from build123d import *

# Parameters (mm, degrees)
F0_W     = 49.7
F0_H     = 1.5
F1_DEPTH = 142
F2_W     = 44.6868650615
F2_H     = 1.5
F3_DEPTH = 1
F4_R     = 0.99999


# Not quite as in the source:
# - a fillet or chamfer is up to 0.001 mm smaller than in the source, because OpenCascade refuses the exact size


with BuildPart() as f1:
    # F0 (on Front) → F1 (new body)
    with BuildSketch(Plane.XZ):
        with Locations((24.85, -0.75)):
            Rectangle(F0_W, F0_H)
        with Locations((-24.85, -0.75)):
            Rectangle(F0_W, F0_H)
        Polygon((49.7, -1.5), (0, -1.5), (0, -3), (50.5, -3), align=None)
        Polygon((0, -3), (0, -1.5), (-49.7, -1.5), (-50.5, -3), align=None)
    extrude(amount=F1_DEPTH)

    # F2 (on face) → F3 (join)
    with BuildSketch(Plane.XY):
        with Locations((-22.3434325308, -130.4639992552)):
            Rectangle(F2_W, F2_H)
        with Locations((22.3434325308, -130.4639992552)):
            Rectangle(F2_W, F2_H)
        with Locations((-22.3434325308, -126.9639992552)):
            Rectangle(F2_W, F2_H)
        with Locations((22.3434325308, -126.9639992552)):
            Rectangle(F2_W, F2_H)
        with Locations((-22.3434325308, -123.4639992552)):
            Rectangle(F2_W, F2_H)
        with Locations((22.3434325308, -123.4639992552)):
            Rectangle(F2_W, F2_H)
    extrude(amount=F3_DEPTH)

    # F4 (radius 1 in the source; OpenCascade refuses exactly that, so slightly less here)
    f4_edges = [f1.edges().sort_by_distance(p)[0] for p in [
        (-44.686865, -123.463999, 1),
        (-44.686865, -126.963999, 1),
        (-44.686865, -130.463999, 1),
        (44.686865, -123.463999, 1),
        (44.686865, -126.963999, 1),
        (44.686865, -130.463999, 1),
        (0, -142, 0),
    ]]
    fillet(f4_edges, radius=F4_R)


solid = f1.part
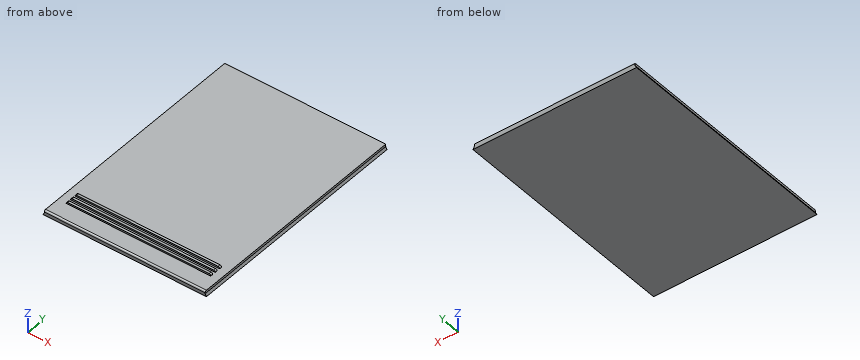
Geometry: final body of the model. Coordinates: model frame, mm. Coordinates: 2 decimals unless noted, no trailing zeros. Order: outer loops, then holes, each group sorted by start corner. A loop starts at its lowest first (then second) coordinate and runs counter-clockwise, first axis right, second up. Notation, with made-up numbers: M 17.25,42 L 72.25,42 A33 cw 72.25,75 Z; hole C 21.25,23.25 d7. An arc over 180 degrees is marked long. One line per question, with ' | ' between items. Start each with the question number.
Item 1: Pin query (flat end, axial travel): pin 1 Ø1.7 at (y, z) = (-79.5, -0.5) entering from -X; pin 2 Ø0.5 at (x, z) = (6.5, 0.5) entering from -Y; pin 3 Ø0.8 at (x, z) = (-6.5, 0.5) entering from +Y. Return the tip coordinate at first contact, or that it passes through.
Item 2: Cut plane B-B, the plane y = -68.5. Return the cut outline in (x, z).
Item 3: Ray query, probe 1 along Y at (x, z) = (25, 0.4); probe 2 along Z at (x, y) = (-19.5, -73.5); probe 3 along X at (y, z) = (-64, -0.9). Return the intervals inside material, ascending. Write a range as [from, to].
Item 4: Cut plane A-A, the plane x = 36.5. Return the cut outline in (y, z), then the cut area to 3 significant figures.
A:
1) pin 1: stops at x = -49.7 | pin 2: stops at y = -131.21 | pin 3: stops at y = -122.71
2) outline: M -50.5,-3 L 50.5,-3 L 49.7,-1.5 L 49.7,0 L -49.7,0 L -49.7,-1.5 Z
3) probe 1: y = [-131.21, -129.71], [-127.71, -126.21], [-124.21, -122.71] | probe 2: z = [-3, 0] | probe 3: x = [-49.7, 49.7]
4) outline: M -142,-3 L 0,-3 L 0,0 L -122.71,0 L -122.71,1 L -124.21,1 L -124.21,0 L -126.21,0 L -126.21,1 L -127.71,1 L -127.71,0 L -129.71,0 L -129.71,1 L -131.21,1 L -131.21,0 L -141,0 A1 ccw -142,-1 Z | area: 430 mm2
